The model under review builds one solid part; all positions refer to its coordinate system, in mm. Face numbers are marked on the shaded views. A direction names the side the tool comes from. Give positions to 0.01 mm unless a question says otherwise; leave off trailing zeros. Loops run counter-clockwise (first coordinate to the right, second up) from the corner with the lowest first, then second, coordinate; pieces in that order, holes last. Notation, with made-up numbers: (67.5, 36) - (90.5, 36) arc R23 ccw to (90.5, 62) - close; hole circle Ø1 at (53.5, 66.5). An arc over 180 degrees is marked (long way). Answer as a JSON object with one key per item and string values.
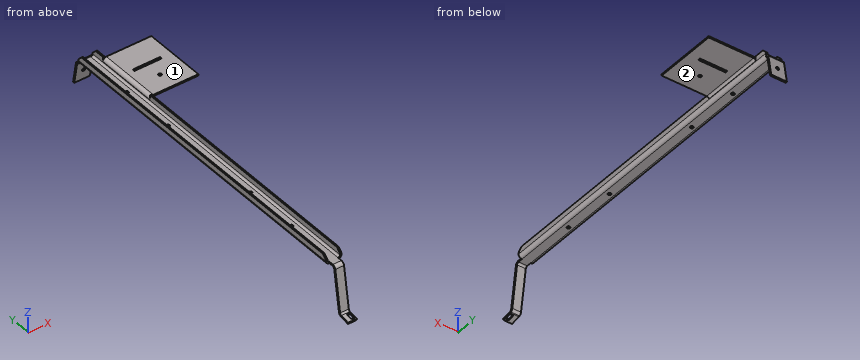
from build123d import *

# Parameters (mm, degrees)
SKETCH1_W                      = 20
SKETCH1_H                      = 425.14614931
BASE_FLANGE1_DEPTH             = 1.89738
EDGE_FLANGE1_START             = 74
EDGE_FLANGE1_DEPTH             = 20
EDGE_FLANGE1_2_DEPTH           = 20
EDGE_FLANGE3_STRIP_W           = 12.66952
EDGE_FLANGE3_STRIP_H           = 1.89738
EDGE_FLANGE3_STRIP_CUT_DEPTH   = 421.088186102
EDGE_FLANGE3_STRIP_2_W         = 12.66952
EDGE_FLANGE3_STRIP_2_H         = 1.89738
EDGE_FLANGE3_STRIP_CUT_2_DEPTH = 421.088186102
EDGE_FLANGE3_DEPTH             = 421.088186102
EDGE_FLANGE3_BEND_DEPTH        = 421.088186102
EDGE_FLANGE5_START             = 78.43738
EDGE_FLANGE5_DEPTH             = 11.12524
EDGE_FLANGE6_START             = 78.43738
EDGE_FLANGE6_DEPTH             = 11.12524
EDGE_FLANGE6_2_DEPTH           = 11.12524
SKETCH31_R                     = 2.04
CUT_EXTRUDE1_DEPTH             = 10
CUT_EXTRUDE2_DEPTH             = 3.21412
BREAK_CORNER1_START            = 74
BREAK_CORNER1_DEPTH            = 20
EDGE_FLANGE7_STRIP_W           = 14.16952
EDGE_FLANGE7_STRIP_H           = 1.89738
EDGE_FLANGE7_STRIP_CUT_DEPTH   = 80
EDGE_FLANGE7_DEPTH             = 80
SKETCH36_W                     = 35
SKETCH36_H                     = 3
CUT_EXTRUDE3_DEPTH             = 10
SKETCH37_R                     = 2.04
CUT_EXTRUDE4_DEPTH             = 10
SKETCH38_R                     = 2.04
CUT_EXTRUDE6_DEPTH             = 10


# Read off the part's stored shape, not the designer's step: Edge-Flange1, Edge-Flange5, Edge-Flange6, Break-Corner1
# Sheet-metal steps are written as plain solids
with BuildPart() as part:
    # Sketch1 → Base-Flange1 (new body)
    with BuildSketch(Plane.XY):
        with Locations((84, -2.062852184)):
            Rectangle(SKETCH1_W, SKETCH1_H)
    extrude(amount=-BASE_FLANGE1_DEPTH)

    # Edge-Flange1 outline → Edge-Flange1 (cut)
    with BuildSketch(Plane.YZ.offset(EDGE_FLANGE1_START)):
        with BuildLine():
            ThreePointArc((206.452259263, 0), (208.504014129, -0.502835143), (210.090767372, -1.89738))
            Line((210.090767372, -1.89738), (210.510222471, -1.89738))
            Line((210.510222471, -1.89738), (210.510222471, 0))
            Line((210.510222471, 0), (206.452259263, 0))
        make_face()
    extrude(amount=EDGE_FLANGE1_DEPTH, mode=Mode.SUBTRACT)

    # Edge-Flange1 2 outline → Edge-Flange1 2 (add)
    with BuildSketch(Plane.YZ.offset(EDGE_FLANGE1_START)):
        with BuildLine():
            Line((215.55374818, -30.500635662), (210.82222549, -3.666837049))
            ThreePointArc((210.82222549, -3.666837049), (210.553071361, -2.742186382), (210.090767372, -1.89738))
            Line((210.090767372, -1.89738), (206.452259263, -1.89738))
            ThreePointArc((206.452259263, -1.89738), (208.084939792, -2.491627114), (208.953670956, -3.996313629))
            Line((208.953670956, -3.996313629), (213.685193646, -30.830112242))
            Line((213.685193646, -30.830112242), (215.55374818, -30.500635662))
        make_face()
    extrude(amount=EDGE_FLANGE1_2_DEPTH)

    # Edge-Flange3 strip (across the edge) → Edge-Flange3 strip cut (cut)
    with BuildSketch(Plane(origin=(74, 206.452259263, 0), x_dir=(1, 0, 0), z_dir=(0, -1, 0))):
        with Locations((-1.89738, -0.94869)):
            Rectangle(EDGE_FLANGE3_STRIP_W, EDGE_FLANGE3_STRIP_H)
    extrude(amount=EDGE_FLANGE3_STRIP_CUT_DEPTH, mode=Mode.SUBTRACT)

    # Edge-Flange3 strip 2 (across the edge) → Edge-Flange3 strip cut 2 (cut)
    with BuildSketch(Plane(origin=(94, -214.635926839, 0), x_dir=(-1, 0, 0), z_dir=(0, 1, 0))):
        with Locations((-1.89738, -0.94869)):
            Rectangle(EDGE_FLANGE3_STRIP_2_W, EDGE_FLANGE3_STRIP_2_H)
    extrude(amount=EDGE_FLANGE3_STRIP_CUT_2_DEPTH, mode=Mode.SUBTRACT)

    # Edge-Flange3 section (across the edge) → Edge-Flange3 (add)
    with BuildSketch(Plane(origin=(74, 206.452259263, 0), x_dir=(1, 0, 0), z_dir=(0, -1, 0))):
        with BuildLine():
            Line((0, 2.54), (0, 9.26))
            Line((0, 9.26), (1.89738, 9.26))
            Line((1.89738, 9.26), (1.89738, 2.54))
            ThreePointArc((1.89738, 2.54), (2.641328776, 0.743948776), (4.43738, 0))
            Line((4.43738, 0), (4.43738, -1.89738))
            ThreePointArc((4.43738, -1.89738), (1.299678511, -0.597701489), (0, 2.54))
        make_face()
    extrude(amount=EDGE_FLANGE3_DEPTH)

    # Edge-Flange3 section 2 (across the edge) → Edge-Flange3 bend (add)
    with BuildSketch(Plane(origin=(94, -214.635926839, 0), x_dir=(-1, 0, 0), z_dir=(0, 1, 0))):
        with BuildLine():
            Line((0, 2.54), (0, 9.26))
            Line((0, 9.26), (1.89738, 9.26))
            Line((1.89738, 9.26), (1.89738, 2.54))
            ThreePointArc((1.89738, 2.54), (2.641328776, 0.743948776), (4.43738, 0))
            Line((4.43738, 0), (4.43738, -1.89738))
            ThreePointArc((4.43738, -1.89738), (1.299678511, -0.597701489), (0, 2.54))
        make_face()
    extrude(amount=EDGE_FLANGE3_BEND_DEPTH)

    # Edge-Flange5 outline → Edge-Flange5 (add)
    with BuildSketch(Plane.YZ.offset(EDGE_FLANGE5_START)):
        with BuildLine():
            ThreePointArc((-220.545530818, 0), (-223.427378599, -1.063169777), (-224.928279306, -3.743220834))
            Line((-224.928279306, -3.743220834), (-233.964581883, -60.796189915))
            Line((-233.964581883, -60.796189915), (-232.090561779, -61.09300554))
            Line((-232.090561779, -61.09300554), (-223.054259203, -4.040036459))
            ThreePointArc((-223.054259203, -4.040036459), (-222.195128861, -2.505948848), (-220.545530818, -1.89738))
            Line((-220.545530818, -1.89738), (-214.635926839, -1.89738))
            Line((-214.635926839, -1.89738), (-214.635926839, 0))
            Line((-214.635926839, 0), (-220.545530818, 0))
        make_face()
    extrude(amount=EDGE_FLANGE5_DEPTH)

    # Edge-Flange6 outline → Edge-Flange6 (cut)
    with BuildSketch(Plane.YZ.offset(EDGE_FLANGE6_START)):
        with BuildLine():
            ThreePointArc((-231.141243496, -55.099245789), (-231.958853079, -57.047079402), (-233.584451669, -58.3961422))
            Line((-233.584451669, -58.3961422), (-233.964581883, -60.796189915))
            Line((-233.964581883, -60.796189915), (-232.090561779, -61.09300554))
            Line((-232.090561779, -61.09300554), (-231.141243496, -55.099245789))
        make_face()
    extrude(amount=EDGE_FLANGE6_DEPTH, mode=Mode.SUBTRACT)

    # Edge-Flange6 2 outline → Edge-Flange6 2 (add)
    with BuildSketch(Plane.YZ.offset(EDGE_FLANGE6_START)):
        with BuildLine():
            Line((-246.408498712, -60.830152569), (-234.753449034, -58.775052849))
            ThreePointArc((-234.753449034, -58.775052849), (-234.155770092, -58.626260643), (-233.584451669, -58.3961422))
            Line((-233.584451669, -58.3961422), (-233.015263599, -54.802430164))
            ThreePointArc((-233.015263599, -54.802430164), (-233.712335844, -56.185396154), (-235.082925613, -56.906498315))
            Line((-235.082925613, -56.906498315), (-246.737975292, -58.961598035))
            Line((-246.737975292, -58.961598035), (-246.408498712, -60.830152569))
        make_face()
    extrude(amount=EDGE_FLANGE6_2_DEPTH)

    # Sketch31 → Cut-Extrude1 (cut)
    with BuildSketch(Plane(origin=(0, 203.838091474, 35.942155223), x_dir=(1, 0, 0), z_dir=(0, 0.9848077530122075, 0.17364817766693413))):
        with Locations(Location((84.110673768, 53.230127546, 0), (0, 0, 270))):
            Circle(SKETCH31_R)
    extrude(amount=-CUT_EXTRUDE1_DEPTH, mode=Mode.SUBTRACT)

    # Sketch32 → Cut-Extrude2 (cut)
    with BuildSketch(Plane(origin=(0, 2.642966784, -14.989009472), x_dir=(1, 0, 0), z_dir=(0, -0.17364817766693053, 0.984807753012208))):
        with BuildLine():
            Line((84.41238, -249.228045081), (84.41238, -244.228045081))
            ThreePointArc((84.41238, -244.228045081), (86.43738, -242.203045081), (88.46238, -244.228045081))
            Line((88.46238, -244.228045081), (88.46238, -249.228045081))
            ThreePointArc((88.46238, -249.228045081), (86.43738, -251.253045081), (84.41238, -249.228045081))
        make_face()
    extrude(amount=-CUT_EXTRUDE2_DEPTH, mode=Mode.SUBTRACT)

    # Break-Corner1 outline → Break-Corner1 (cut)
    with BuildSketch(Plane.YZ.offset(BREAK_CORNER1_START)):
        Polygon((-214.635926839, 9.26), (-214.635926839, 4.26), (-209.635926839, 9.26), align=None)
        Polygon((206.452259263, 9.26), (201.452259263, 9.26), (206.452259263, 4.26), align=None)
    extrude(amount=BREAK_CORNER1_DEPTH, mode=Mode.SUBTRACT)

    # Edge-Flange7 strip (across the edge) → Edge-Flange7 strip cut (cut)
    with BuildSketch(Plane(origin=(94, 189.043786616, 7.76), x_dir=(0, 0, -1), z_dir=(0, -1, 0))):
        with Locations((-2.64738, -0.94869)):
            Rectangle(EDGE_FLANGE7_STRIP_W, EDGE_FLANGE7_STRIP_H)
    extrude(amount=EDGE_FLANGE7_STRIP_CUT_DEPTH, mode=Mode.SUBTRACT)

    # Edge-Flange7 section (across the edge) → Edge-Flange7 (add)
    with BuildSketch(Plane(origin=(94, 189.043786616, 7.76), x_dir=(0, 0, -1), z_dir=(0, -1, 0))):
        with BuildLine():
            Line((0, 2.54), (0, 60))
            Line((0, 60), (1.89738, 60))
            Line((1.89738, 60), (1.89738, 2.54))
            ThreePointArc((1.89738, 2.54), (2.641328776, 0.743948776), (4.43738, 0))
            Line((4.43738, 0), (4.43738, -1.89738))
            ThreePointArc((4.43738, -1.89738), (1.299678511, -0.597701489), (0, 2.54))
        make_face()
    extrude(amount=EDGE_FLANGE7_DEPTH)

    # Sketch36 → Cut-Extrude3 (cut)
    with BuildSketch(Plane.XY.offset(7.76)):
        with Locations((122.44, 154.043786616)):
            Rectangle(SKETCH36_W, SKETCH36_H)
    extrude(amount=-CUT_EXTRUDE3_DEPTH, mode=Mode.SUBTRACT)

    # Sketch37 → Cut-Extrude4 (cut)
    with BuildSketch(Plane.XY):
        with Locations((83.43738, 136.452259263)):
            Circle(SKETCH37_R)
        with Locations((83.43738, 66.452259263)):
            Circle(SKETCH37_R)
        with Locations((83.43738, -73.547740737)):
            Circle(SKETCH37_R)
        with Locations((83.43738, -143.547740737)):
            Circle(SKETCH37_R)
    extrude(amount=-CUT_EXTRUDE4_DEPTH, mode=Mode.SUBTRACT)

    # Sketch38 → Cut-Extrude6 (cut)
    with BuildSketch(Plane.XY.offset(7.76)):
        with Locations((122.195161073, 132.04291448)):
            Circle(SKETCH38_R)
    extrude(amount=-CUT_EXTRUDE6_DEPTH, mode=Mode.SUBTRACT)


solid = part.part
Q1. To check wall thickness, follow probe 1 along Z at (x, y) = (88, 180.5); probe 2 along Y at (x, z) = (81.5, -23); probe 3 along Y at (x, z) = (88, -3). State the ranges of each line that lie inside material, in increasing order. Write a range as [from, to].
Results:
{"probe 1": "z = [-1.9, 0]", "probe 2": "y = [-227.98, -226.06], [212.3, 214.23]", "probe 3": "y = [-224.74, -222.64], [208.55, 210.65]"}
Q2. Consider section A-A, the plane x = 116. State the section outline as (y, z) points, plus the area to 3 significant figures.
Results:
{"outline": "(109.04, 5.86) - (152.54, 5.86) - (152.54, 7.76) - (109.04, 7.76) - close; (155.54, 5.86) - (189.04, 5.86) - (189.04, 7.76) - (155.54, 7.76) - close", "area": "146 mm^2"}
Q3. Clearance check with flat-ended pins moving along their axes: pin 1 Ø3.5 at (x, y) = (83.44, 66.45) entering from +Z; pin 2 Ø9 at (x, y) = (86, -112) entering from +Z; pin 3 Ø0.6 at (x, z) = (124.5, 6.5) entering from -Y; pin 4 Ø3.5 at (x, z) = (76, 1) entering from -Y. State where each tip first meets the part, or that it passes through.
Results:
{"pin 1": "passes through", "pin 2": "stops at z = 0.18", "pin 3": "stops at y = 109.04", "pin 4": "stops at y = -214.64"}
Q4. Consider section D-D, the plane y = 115.5. State the section outline as (x, z) points, plus the area to 3 significant figures.
Results:
{"outline": "(74, 2.54) arc R4.44 ccw to (78.44, -1.9) - (89.56, -1.9) arc R4.44 ccw to (94, 2.54) - (94, 3.32) arc R2.54 cw to (96.54, 5.86) - (154, 5.86) - (154, 7.76) - (96.54, 7.76) arc R4.44 ccw to (92.1, 3.32) - (92.1, 2.54) arc R2.54 cw to (89.56, 0) - (78.44, 0) arc R2.54 cw to (75.9, 2.54) - (75.9, 9.26) - (74, 9.26) - close", "area": "176 mm^2"}
Q5. Consider section B-B, the plane z = -26.5. State the section outline as (x, y) points, plus the area to 3 significant figures.
Results:
{"outline": "(74, 212.92) - (94, 212.92) - (94, 214.85) - (74, 214.85) - close; (78.44, -228.53) - (89.56, -228.53) - (89.56, -226.61) - (78.44, -226.61) - close", "area": "59.9 mm^2"}
Q6. For the marked faces 1 and 2, list the 3-axis set-ups (+Z, -Z, +X, -X, +Y, -Y) from which the entire face can be reached by the end or side of a thin tool; tool diameter is ignored.
Results:
{"face 1": "+Z, +X, +Y, -Y", "face 2": "-Z, +X, +Y, -Y"}
Q7. Consider section C-C, the plane y = 0.5. State the section outline as (x, z) points, plus the area to 3 significant figures.
Results:
{"outline": "(74, 2.54) arc R4.44 ccw to (78.44, -1.9) - (89.56, -1.9) arc R4.44 ccw to (94, 2.54) - (94, 9.26) - (92.1, 9.26) - (92.1, 2.54) arc R2.54 cw to (89.56, 0) - (78.44, 0) arc R2.54 cw to (75.9, 2.54) - (75.9, 9.26) - (74, 9.26) - close", "area": "67.4 mm^2"}
